Verification items for the finished model (mm, model axes). A direction names the side the tool comes from. Coordinates: 2 decimals unless noted, no trailing zeros. Order: outer loops, then holes, each group sorted by start corner. A loop starts at its lowest first (then second) coordinate and runs counter-clockwise, first axis right, second up. Notation, with made-up numbers: (76, 35) -> (104, 35) arc R17 ccw to (104, 66) -> close; hole circle Ø2 at (15.25, 79). An arc over 180 degrees is marked (long way). Answer as CSV lines item,"result".
```python
from build123d import *

# Parameters (mm, degrees)
SKETCH1_W           = 6
SKETCH1_H           = 3
BOSS_EXTRUDE2_DEPTH = 3


with BuildPart() as part:
    # Sketch1 → Boss-Extrude2 (new body)
    with BuildSketch(Plane(origin=(0, 0, 0), x_dir=(1, 0, 0), z_dir=(0, 1, 0))):
        Polygon((-57.5, 30), (-82.5, 30), (-82.5, 5), (-79.5, 5), (-79.5, -5), (-82.5, -5), (-82.5, -30), (-57.5, -30), (-57.5, -27), (-32.5, -27), (-32.5, -30), (32.5, -30), (32.5, -27), (57.5, -27), (57.5, -30), (82.5, -30), (82.5, -5), (79.5, -5), (79.5, 5), (82.5, 5), (82.5, 30), (57.5, 30), (57.5, 27), (32.5, 27), (32.5, 30), (-32.5, 30), (-32.5, 27), (-57.5, 27), align=None)
        with Locations((0, -25.5)):
            Rectangle(SKETCH1_W, SKETCH1_H, mode=Mode.SUBTRACT)
    extrude(amount=BOSS_EXTRUDE2_DEPTH)


solid = part.part
```
Item 1: Tool access check on faces 5 (the flat face through (45, 1, 27)), 6 (the flat face through (-3, 1, 26)), 7 (the flat face through (81, 1, -5)), 8 (the flat face through (32.5, 1, -28)). Record the directions out of +Z, -Z, +X, -X, +Y, -Y that give a thin tool (end or side, any length) a straight path to the whole face; none if there is none.
Answer list:
face 5,"+Z, +Y, -Y"
face 6,"+Y, -Y"
face 7,"+X, +Y, -Y"
face 8,"-Z, +Y, -Y"
Item 2: Section check D-D, the plane z = 2. Record the boundary of the cut face in (x, y).
Answer list:
outline,"(-79.5, 0) -> (79.5, 0) -> (79.5, 3) -> (-79.5, 3) -> close"
Item 3: Release check for a two-part mould opening along X. For faces 1 (the flat face through (81, 1, 5)), 2 (the flat face through (57.5, 1, 28)), 3 (the flat face through (-45, 1, -27)), 4 (the flat face through (-79.5, 1, 0)) record: +X half, -X half, draft (parallel to the pull), parting line (faces both ways), or undercut.
Answer list:
face 1,"draft"
face 2,"undercut"
face 3,"undercut"
face 4,"-X half"
Item 4: Thickness scan on line 1 (X direction, y = 0.95, z = 3); line 2 (Z direction, x = 50, y = 1). Record the ranges inside material, lowest first.
Answer list:
line 1,"-79.5 to 79.5"
line 2,"-27 to 27"
Item 5: Depth check by flat-ended pin: pin 1 Ø1.5 at (y, z) = (1.5, 1) entering from +X; pin 2 Ø0.9 at (x, y) = (-45, 1) entering from +Z. Enter the tip coordinate at first touch or a pass-through.
Answer list:
pin 1,"x = 79.5"
pin 2,"z = 27"
Item 6: Section check A-A, the plane z = 25.5. Record the boundary of the cut face in (x, y), plus the area to 3 significant figures.
Answer list:
outline,"(-82.5, 0) -> (-3, 0) -> (-3, 3) -> (-82.5, 3) -> close; (3, 0) -> (82.5, 0) -> (82.5, 3) -> (3, 3) -> close"
area,"477 mm2"
Item 7: Section check C-C, the plane x = -51.5. Record the boundary of the cut face in (y, z).
Answer list:
outline,"(0, -27) -> (3, -27) -> (3, 27) -> (0, 27) -> close"
